Autodesk Inventor part; units mm, degrees
ref_plane "MSC_PF1" through (0, 0, 0) normal (1, 0, 0) x (0, 1, 0)
ref_plane "MSC_PT1" through (0, 0, 0) normal (0, 0, -1) x (-1, 0, 0)
ref_plane "YZ Plane" through (0, 0, 0) normal (1, 0, 0) x (0, 1, 0)
sketch "Эскиз1" plane through (0, 0, 0) normal (0, 1, 0) x (-1, 0, 0)
  point P0 (0, 0)
sketch "Эскиз2" plane through (0, 0, 0) normal (0, 1, 0) x (-1, 0, 0)
  line L0 (-2.5, -10) -> (0, -10)
  line L1 (-2.5, -2.8) -> (-2.5, -10)
  line L2 (-5, -0.3) -> (-2.5, -2.8)
  line L3 (-5, 0) -> (-5, -0.3)
  line L4 (0, 0) -> (-5, 0)
  line L5 (0, -10) -> (0, 0)
  line L6 (0, -10) -> (0, 0)
  line L7 (0, -12) -> (0, 2)
  line L8 (1, 0) -> (-6, 0)
  dimension "d3" = 5
  dimension "d5" = 2.5
  dimension "d7" = 10
  dimension "ParC" = 0.3
  dimension "d22" = 0
  dimension "d23" = 0
  dimension "d43" = 45
revolve "Вращение1" add sketch "Эскиз2" angle 360 about axis through (0, 0, -10) along (0, 0, -1)
sketch "Эскиз3" plane through (0, 0, 0) normal (0, 0, 1) x (1, 0, 0)
  line L0 (-1.5, 0.866) -> (-1.5, -0.866)
  line L1 (0, 1.7321) -> (-1.5, 0.866)
  line L2 (1.5, 0.866) -> (0, 1.7321)
  line L3 (1.5, -0.866) -> (1.5, 0.866)
  line L4 (0, -1.7321) -> (1.5, -0.866)
  line L5 (-1.5, -0.866) -> (0, -1.7321)
  circle A0 centre (0, 0) radius 1.5 construction
  circle A1 centre (0, 0) radius 2.5 construction
  dimension "d11" = 3
  dimension "d13" = 120
  dimension "d15" = 120
extrude "Выдавливание1" cut sketch "Эскиз3" against normal blind 2.3
fillet "Сопряжение1" radius 0.2 1 edges at (-2.5, 0, -2.8)
chamfer "Фаска1" distance 0.4 angle 45 1 edges at (-2.5, 0, -10) measured on face at (-0.599, -2.4272, -7.6276)
thread "Резьба1"
ref_plane "MSC_PF1" through (0, 0, 0) normal (1, 0, 0) x (0, 1, 0)
ref_plane "MSC_PT1" through (0, 0, 0) normal (0, 0, -1) x (-1, 0, 0)
equation "\"d3\" = 0.5 * dk"
equation "\"d5\" = 0.5 * NND"
equation "\"d7\" = NLG"
equation "\"d43\" = 0.5 * ang"
equation "\"d11\" = ParS"
equation "\"d16\" = ParT"
equation "\"d18\" = r"
equation "\"d19\" = 0.5 * PTC"
equation "\"d39\" = 0.5 * PTC"
equation "\"NND\" = 5"
equation "\"PTC\" = 0.8"
equation "\"ParK\" = 2.8"
equation "\"ParS\" = 3"
equation "\"ParT\" = 2.3"
equation "\"r\" = 0.2"
equation "\"NLG\" = 10"
equation "\"ang\" = 90deg"
equation "\"THREADDIA\" = NND"
properties part number "DIN 7991 - M5x10" material "Сталь, мягкая"
Design review of the part built by this model. Coordinates are the model's own, in mm. A direction names the side the tool comes from. Coordinates: 2 decimals unless noted, no trailing zeros. Order: outer loops, then holes, each group sorted by start corner. A loop starts at its lowest first (then second) coordinate and runs counter-clockwise, first axis right, second up. Notation, with made-up numbers: (65.25, 89) -> (107.25, 89) arc R29 cw to (107.25, 119) -> close; hole circle Ø4 at (-8, 60.5). An arc over 180 degrees is marked (long way). One line per item, written item: value.
1) Clearance check with flat-ended pins moving along their axes: P1, Ø1.5, axis at x = 2.5, y = 4, coming from the -Z side; P2, Ø3, axis at y = -0.5, z = -9, coming from the +X side; P3, Ø0.9, axis at y = 0.5, z = -1, coming from the -X side. State where each tip first meets the part, or that it passes through.
Output values:
P1: stops at z = -1.33
P2: stops at x = 2.5
P3: stops at x = -4.73
2) We need section A-A, the plane z = -5.75. Give the boundary of the cut face in (x, y).
Output values:
outline: circle Ø5 at (0, 0)
3) To check wall thickness, follow probe 1 along X at (y, z) = (0, -9); probe 2 along Z at (x, y) = (-2.75, -0.5); probe 3 along X at (y, z) = (-1.25, -1). State the ranges of each line that lie inside material, in increasing order. Write a range as [from, to].
Output values:
probe 1: x = [-2.5, 2.5]
probe 2: z = [-2.5, 0]
probe 3: x = [-4.11, -0.83], [0.83, 4.11]
4) Draft analysis for pull direction X (two halves, no side actions). For faces 4 (the face through (0, 0, -2.3)), 5 (the face through (2, 0, 0)), 6 (the face through (-0.74, 1.305, -1.134)), 7 (the face through (4.77, -1.5, -0.15)), state which applies: +X half, -X half, draft (parallel to the pull), parting line (faces both ways), or undercut.
Output values:
face 4: undercut
face 5: draft
face 6: undercut
face 7: parting line
5) Machinability: for faces 1 (the face through (-0.54, 2.44, -6.29)), 2 (the face through (0, 0, -10)), 3 (the face through (0.76, 1.293, -1.134)), which of the approach directions +Z, -Z, +X, -X, +Y, -Y give a long, thin tool a straight path to every point of the face, cutting with its end or side? Answer none if there is none.
Output values:
face 1: -Z
face 2: -Z, +X, -X, +Y, -Y
face 3: +Z
